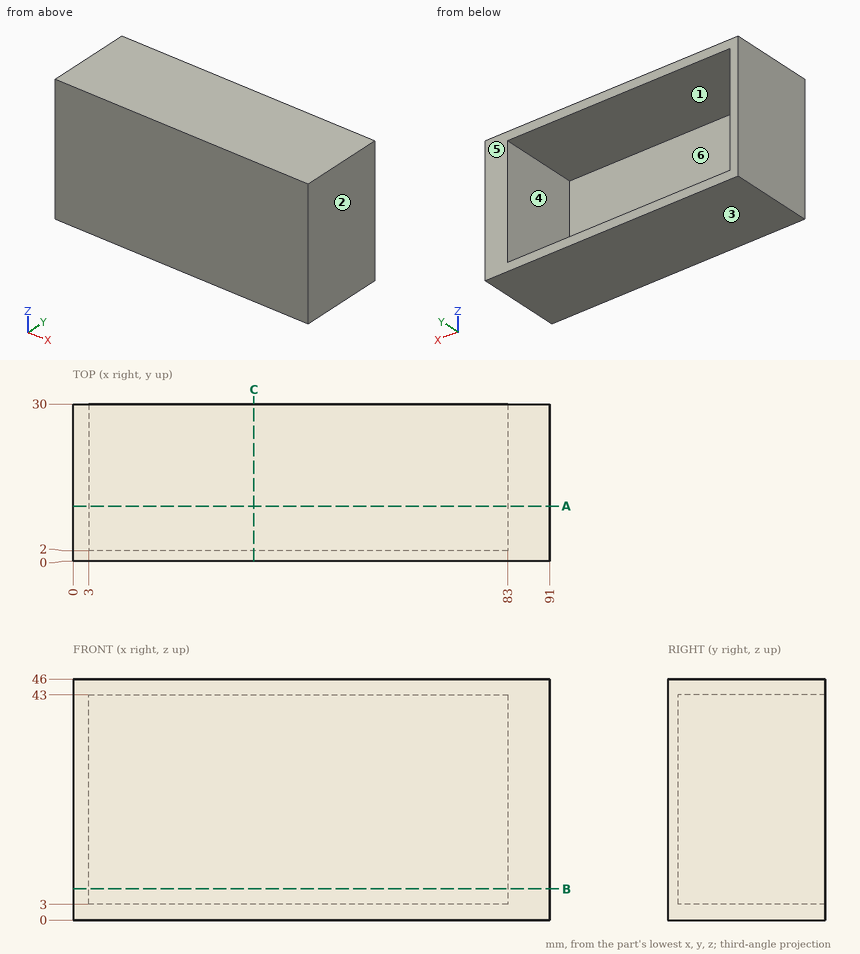
Geometry: see drawing. Coordinates: mm, zero at the bounding-box minimum. A direction names the side the tool comes from. Give positions to 0.01 mm unless a question says otherwise; leave off trailing zeros. Loops run counter-clockwise (first coordinate to the right, second up) from the corner with the lowest first, then second, coordinate; pieces in that order, holes last. Notation, with made-up numbers: (65.5, 17) - (106.5, 17) arc R31 ccw to (106.5, 55) - close; hole circle Ø9 at (24.5, 1). An arc over 180 degrees is marked (long way). Use CSV: the item, a comma, the result in double quotes.
1) Cut plane C-C (x = 34.5). Output: boundary loops of the cut face in (y, z), and give its area (3 significant figures).
Worked out:
outline,"(0, 0) - (30, 0) - (30, 3) - (2, 3) - (2, 43) - (30, 43) - (30, 46) - (0, 46) - close"
area,"260 mm^2"
2) Cut plane A-A (y = 10.5). Output: boundary loops of the cut face in (x, z), and give its area (3 significant figures).
Worked out:
outline,"(0, 0) - (91, 0) - (91, 46) - (0, 46) - close; hole (3, 3) - (83, 3) - (83, 43) - (3, 43) - close"
area,"986 mm^2"
3) Set-up query: the marked faces 1 and 2. Return all of +Z, -Z, +X, -X, +Y, -Y with unobstructed straight access to the full face (end or side cutting, diameter ignored); none if empty.
Worked out:
face 1,"+Y"
face 2,"+Z, -Z, +X, +Y, -Y"
4) Cut plane B-B (z = 6). Output: boundary loops of the cut face in (x, y).
Worked out:
outline,"(0, 0) - (91, 0) - (91, 30) - (83, 30) - (83, 2) - (3, 2) - (3, 30) - (0, 30) - close"
5) Pin query (flat end, axial travel): P1, Ø8, axis at x = 77.5, y = 17.5, coming from the -Z side; P2, Ø3, axis at x = 11, z = 22.5, coming from the +Y side. Return the tip coordinate at first contact, or that it passes through.
Worked out:
P1,"stops at z = 0"
P2,"stops at y = 2"
6) Mould query, pull axis Z, two halves, no side actions, for the marked faces 3, 4, 5 and 6. Classes: +Z half, -Z half, draft (parallel to the pull), parting line (faces both ways), or undercut.
Worked out:
face 3,"-Z half"
face 4,"undercut"
face 5,"draft"
face 6,"undercut"
7) Line query: line 1 (X direction, y = 20.75, z = 31); line 2 (Z direction, x = 24, y = 7.5); line 3 (Y direction, x = 29, z = 28.5). Output: solid intervals per line, ascending.
Worked out:
line 1,"x = 0 to 3, 83 to 91"
line 2,"z = 0 to 3, 43 to 46"
line 3,"y = 0 to 2"
